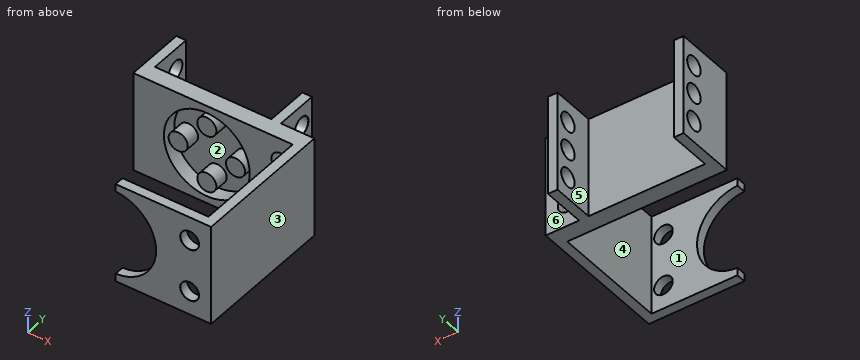
from build123d import *

# Parameters (mm, degrees)
BOSS_EXTRUDE1_DEPTH              = 21
M3_5_CLEARANCE_HOLE1_D           = 3.9
M3_5_CLEARANCE_HOLE1_CSINK_D     = 3.95
M3_5_CLEARANCE_HOLE1_CSINK_ANGLE = 90
SKETCH4_R                        = 9
SKETCH4_R_2                      = 2
CUT_EXTRUDE1_DEPTH               = 3
SKETCH5_R                        = 8.9
CUT_EXTRUDE2_DEPTH               = 3
M3_5_CLEARANCE_HOLE2_D           = 3.9
M3_5_CLEARANCE_HOLE2_CSINK_D     = 3.95
M3_5_CLEARANCE_HOLE2_CSINK_ANGLE = 90


with BuildPart() as part:
    # Sketch1 → Boss-Extrude1 (new body)
    with BuildSketch(Plane.XY):
        Polygon((14.42095576, -30), (21.42095576, -30), (21.42095576, -59.9), (1.42095576, -59.9), (1.42095576, -57.9), (19.42095576, -57.9), (19.42095576, -33.5), (14.42095576, -33.5), (-13.97904424, -33.5), (-13.97904424, -21), (-11.97904424, -21), (-11.97904424, -30), (12.42095576, -30), (12.42095576, -21), (14.42095576, -21), align=None)
    extrude(amount=-BOSS_EXTRUDE1_DEPTH)

    # M3.5 Clearance Hole1 (through all)
    with Locations(Plane(origin=(14.42095576, 0, 0), x_dir=(0, 0, -1), z_dir=(1, 0, 0))):
        with Locations((4.5, -24), (10.5, -24), (16.5, -24)):
            CounterSinkHole(M3_5_CLEARANCE_HOLE1_D / 2, M3_5_CLEARANCE_HOLE1_CSINK_D / 2, counter_sink_angle=M3_5_CLEARANCE_HOLE1_CSINK_ANGLE)

    # Sketch4 → Cut-Extrude1 (cut)
    with BuildSketch(Plane.XZ.offset(33.5)):
        with Locations((1.42095576, -10.5)):
            Circle(SKETCH4_R)
        with Locations((1.42095576, -4.5)):
            Circle(SKETCH4_R_2, mode=Mode.SUBTRACT)
        with Locations((1.42095576, -16.5)):
            Circle(SKETCH4_R_2, mode=Mode.SUBTRACT)
        with Locations((-4.57904424, -10.5)):
            Circle(SKETCH4_R_2, mode=Mode.SUBTRACT)
        with Locations((7.42095576, -10.5)):
            Circle(SKETCH4_R_2, mode=Mode.SUBTRACT)
    extrude(amount=-CUT_EXTRUDE1_DEPTH, mode=Mode.SUBTRACT)

    # Sketch5 → Cut-Extrude2 (cut)
    with BuildSketch(Plane.XZ.offset(59.9)):
        with Locations((0.99475454, -10.484843567)):
            Circle(SKETCH5_R)
    extrude(amount=-CUT_EXTRUDE2_DEPTH, mode=Mode.SUBTRACT)

    # M3.5 Clearance Hole2 (through all)
    with Locations(Plane(origin=(0, -59.9, 0), x_dir=(-1, 0, 0), z_dir=(0, -1, 0))):
        with Locations((-16.92095576, 16), (-16.92095576, 5)):
            CounterSinkHole(M3_5_CLEARANCE_HOLE2_D / 2, M3_5_CLEARANCE_HOLE2_CSINK_D / 2, counter_sink_angle=M3_5_CLEARANCE_HOLE2_CSINK_ANGLE)


solid = part.part
Geometry: final body of the model. Coordinates: model frame, mm. Face numbers are marked on the shaded views. A direction names the side the tool comes from. Give positions to 0.01 mm unless a question says otherwise; leave off trailing zeros. Order: outer loops, then holes, each group sorted by start corner. A loop starts at its lowest first (then second) coordinate and runs counter-clockwise, first axis right, second up. Notation, with made-up numbers: (53, -20) - (91, -20) arc R4 ccw to (91, -16) - close; hole circle Ø4 at (37.25, 33.25). An arc over 180 degrees is marked (long way). Use CSV: the item, a comma, the result in double quotes.
1. Section query C-C (y = -24). Give the number of separate pieces and of enclosed holes in the cut face, plus the area to 3 significant figures.
Answers below:
separate pieces,"8"
enclosed holes,"0"
area,"37.2 mm2"
2. Mould query, pull axis X, two halves, no side actions, for the marked faces 1, 2 and 3. Classes: +X half, -X half, draft (parallel to the pull), parting line (faces both ways), or undercut.
Answers below:
face 1,"draft"
face 2,"undercut"
face 3,"+X half"
3. Access query for the marked faces 4, 5 and 6. Directions: +Z, -Z, +X, -X, +Y, -Y. A direction counts if a zero-diameter tool reaches every point of the face in a straight line with its end or side. Return the directions, or none.
Answers below:
face 4,"+Z, -Z, -X"
face 5,"+Z, -Z, +Y"
face 6,"+Z, -Z, +X, +Y"
4. Section query B-B (x = 7.5). Output: boundary loops of the cut face in (y, z).
Answers below:
outline,"(-59.9, -21) - (-57.9, -21) - (-57.9, -16.56) - (-59.9, -16.56) - close; (-59.9, -4.41) - (-57.9, -4.41) - (-57.9, 0) - (-59.9, 0) - close; (-33.5, -21) - (-30, -21) - (-30, 0) - (-33.5, 0) - (-33.5, -3.86) - (-30.5, -3.86) - (-30.5, -8.5) - (-33.5, -8.5) - (-33.5, -12.5) - (-30.5, -12.5) - (-30.5, -17.14) - (-33.5, -17.14) - close"
5. Material intervals for line 1 along Y through (x, z) = (13.5, -10.5); line 2 along Y through (x, z) = (-12.7, -10.5); line 3 along X through (y, z) = (-24.5, -13), sorted ascending. Write a range as from..to.
Answers below:
line 1,"-59.9..-57.9, -33.5..-25.95, -22.05..-21"
line 2,"-33.5..-25.95, -22.05..-21"
line 3,"-13.98..-11.98, 12.42..14.42"
6. Section query A-A (y = -28). Output: boundary loops of the cut face in (x, z), plus the area to 3 significant figures.
Answers below:
outline,"(-13.98, -21) - (-11.98, -21) - (-11.98, 0) - (-13.98, 0) - close; (12.42, -21) - (14.42, -21) - (14.42, 0) - (12.42, 0) - close"
area,"84.0 mm2"
7. Contact query for flat-ended pins moving along their axis: pin 1 (1.8 mm diameter, centred on y = -59, z = -0.5, fed in from -X); pin 2 (5 mm diameter, centred on y = -44, z = -7.5, fed in from -X); pin 3 (1.2 mm diameter, centred on x = 1.5, z = -17, fed in from -Y). Output: stop coordinate, or through.
Answers below:
pin 1,"x = 1.42"
pin 2,"x = 19.42"
pin 3,"y = -33.5"
